Geometry check sheet. Reference: the model listing, model coordinates, mm. A direction names the side the tool comes from. Round coordinates to 2 decimals unless told otherwise and drop trailing zeros. Loops run counter-clockwise (first coordinate to the right, second up) from the corner with the lowest first, then second, coordinate; pieces in that order, holes last. Notation, with made-up numbers: (-28.75, 89) -> (5.25, 89) arc R14 cw to (5.25, 95) -> close; hole circle Ø3 at (69.25, 13). An arc over 180 degrees is marked (long way). Use one line per item in the form item = value.
from build123d import *

# Parameters (mm, degrees)
F1_DEPTH = 63.5
F0_W     = 11.7803301271
F0_H     = 19.05
F2_DEPTH = 25.4
F3_DEPTH = 7.9375
F4_R     = 6.35


with BuildPart() as f1:
    # F0 (on Front) → F1 (new body, symmetric)
    with BuildSketch(Plane.XZ):
        Polygon((41.275, -9.525), (41.275, 9.525), (22.225, 9.525), (-41.275, 9.525), (-41.275, -9.525), align=None)
    extrude(amount=F1_DEPTH, both=True)

    # F0 (on Front) → F2 (join, symmetric)
    with BuildSketch(Plane.XZ):
        with BuildLine():
            Line((22.225, 9.525), (41.275, 9.525))
            Line((41.275, 9.525), (41.275, 27.0178999029))
            ThreePointArc((41.275, 27.0178999029), (45.6627686716, 37.9750501441), (56.4005611221, 42.8752))
            Line((56.4005611221, 42.8752), (61.7728, 42.8752))
            Line((61.7728, 42.8752), (61.7728, 61.9252))
            Line((61.7728, 61.9252), (56.0382334177, 61.9252))
            ThreePointArc((56.0382334177, 61.9252), (32.0643061399, 51.3173564515), (22.225, 27.0178999029))
            Line((22.225, 27.0178999029), (22.225, 9.525))
        make_face()
        Polygon((87.1728, 52.3875), (87.1728, 38.1), (112.5728, 38.1), (112.5728, 66.675), (87.1728, 66.675), align=None)
        Polygon((73.5531301271, 42.8752), (61.7728, 42.8752), (61.7728, 38.1), (87.1728, 38.1), (87.1728, 52.3875), (87.1728, 66.675), (61.7728, 66.675), (61.7728, 61.9252), (73.5531301271, 61.9252), align=None)
        with Locations((67.6629650635, 52.4002)):
            Rectangle(F0_W, F0_H)
    extrude(amount=F2_DEPTH, both=True)

    # F0 (on Front) → F3 (join, symmetric)
    with BuildSketch(Plane.XZ):
        with BuildLine():
            Line((-41.275, 9.525), (22.225, 9.525))
            Line((22.225, 9.525), (22.225, 27.0178999029))
            ThreePointArc((22.225, 27.0178999029), (32.0643061399, 51.3173564515), (56.0382334177, 61.9252))
            add(Edge.make_bspline(
                [(-41.275, 9.525), (-23.4800241888, 55.0344586372), (8.1693455577, 62.4129325151), (56.0382334177, 61.9252)],
                knots=[0, 0, 0, 0, 110.5244152133, 110.5244152133, 110.5244152133, 110.5244152133], degree=3))
        make_face()
    extrude(amount=F3_DEPTH, both=True)

    # F4
    f4_edges = [f1.edges().sort_by_distance(p)[0] for p in [
        (41.275, -63.5, 0),
        (41.275, 63.5, 0),
        (-41.275, -63.5, 0),
        (-41.275, 63.5, 0),
    ]]
    fillet(f4_edges, radius=F4_R)


solid = f1.part
1. Section check A-A (z = 6). Record the boundary of the cut face in (x, y) (3 decimals).
Return value:
outline = (-41.275, -57.15) arc R6.35 ccw to (-34.925, -63.5) -> (34.925, -63.5) arc R6.35 ccw to (41.275, -57.15) -> (41.275, 57.15) arc R6.35 ccw to (34.925, 63.5) -> (-34.925, 63.5) arc R6.35 ccw to (-41.275, 57.15) -> close
2. Tool access check on faces 1 (the cylindrical face through (32.33, 16.55, 51.59)), 2 (the flat face through (67, 25.4, 45)), 3 (the flat face through (87, 0, 38.1)), 4 (the flat face through (67, -25.4, 45)), 5 (the flat face through (61.773, 0, 64)). Record the directions out of +Z, -Z, +X, -X, +Y, -Y that give a thin tool (end or side, any length) a straight path to the whole face; none if there is none.
Return value:
face_1 = +Z, -X, +Y
face_2 = +Z, +X, -X, +Y
face_3 = -Z, +X, +Y, -Y
face_4 = +Z, +X, -X, -Y
face_5 = +Z, -X, +Y, -Y
3. Mould release check, pull along X, two halves, no side actions. Record for faces 6 (the cylindrical face through (32.33, -16.79, 51.59)), 7 (the flat face through (-4, -7.938, 30)), 8 (the flat face through (59, 0, 42.875)): released by +X, released by -X, zero draft, split by the parting line, or undercut.
Return value:
face_6 = released by -X
face_7 = zero draft
face_8 = undercut
4. Material ranges on line 1 along Z through (x, y) = (-3, -17) (3 decimals); line 2 along Y through (x, z) = (41, 40.5); line 3 along X through (y, z) = (8.5, 2) (3 decimals), recorded low to high.
Return value:
line_1 = -9.525 to 9.525
line_2 = -25.4 to 25.4
line_3 = -41.275 to 41.275
5. Section check B-B (y = -11). Record the boundary of the cut face in (x, z) (3 decimals), then the cut area to 3 significant figures.
Return value:
outline = (-41.275, -9.525) -> (41.275, -9.525) -> (41.275, 27.018) arc R15.875 cw to (56.401, 42.875) -> (61.773, 42.875) -> (61.773, 38.1) -> (112.573, 38.1) -> (112.573, 66.675) -> (61.773, 66.675) -> (61.773, 61.925) -> (56.038, 61.925) arc R34.925 ccw to (22.225, 27.018) -> (22.225, 9.525) -> (-41.275, 9.525) -> close
area = 4,210 mm2
6. Section check D-D (y = -39.5). Record the boundary of the cut face in (x, z) (3 decimals), then the cut area to 3 significant figures.
Return value:
outline = (-41.275, -9.525) -> (41.275, -9.525) -> (41.275, 9.525) -> (-41.275, 9.525) -> close
area = 1,570 mm2
7. Section check C-C (x = 98). Record the boundary of the cut face in (y, z) (3 decimals), then the cut area to 3 significant figures.
Return value:
outline = (-25.4, 38.1) -> (25.4, 38.1) -> (25.4, 66.675) -> (-25.4, 66.675) -> close
area = 1,450 mm2
8. Gauge pin test, flat ends, axial feed: pin 1 (15.5 mm diameter, centred on x = 31.5, z = 31.5, fed in from -Y); pin 2 (3 mm diameter, centred on x = 59, y = 0.5, fed in from +Z); pin 3 (2 mm diameter, centred on x = 35.5, z = 44, fed in from +Y). Record the tip position at first contact, or that the pin passes through.
Return value:
pin_1 = -25.4
pin_2 = 61.93
pin_3 = 25.4
